```python
from build123d import *

# Parameters (mm, degrees)
CUT_EXTRUDE1_DEPTH      = 173.110429667
CUT_EXTRUDE1_DEPTH_BACK = 12.7
SKETCH2_W               = 15.5
SKETCH2_H               = 15.5


with BuildPart() as part:
    # Sketch1 → Revolve1 (revolve)
    with BuildSketch(Plane.XY, mode=Mode.PRIVATE) as revolve1_sk:
        Polygon((0, 0), (170, 0), (170, 16), (12.7, 19), (0, 19), align=None)
    revolve(revolve1_sk.sketch.rotate(Axis((0, 0, 0), (1, 0, 0)), 90), axis=Axis((0, 0, 0), (1, 0, 0)))

    # Sketch2 → Cut-Extrude1 (cut, two sides: drawn at the far end of the back side and taken through both)
    with BuildSketch(Plane(origin=(170, 0, 0), x_dir=(0, 0, -1), z_dir=(1, 0, 0)).offset(-CUT_EXTRUDE1_DEPTH_BACK)):
        Rectangle(SKETCH2_W, SKETCH2_H)
    extrude(amount=CUT_EXTRUDE1_DEPTH + CUT_EXTRUDE1_DEPTH_BACK, mode=Mode.SUBTRACT)


solid = part.part
```
Here's how the part is built. I have some questions about the finished solid (model axes, mm). A direction names the side the tool comes from. Give positions to 0.01 mm unless a question says otherwise; leave off trailing zeros. Loops run counter-clockwise (first coordinate to the right, second up) from the corner with the lowest first, then second, coordinate; pieces in that order, holes last. Notation, with made-up numbers: M 52,62.25 L 65,62.25 A25 ccw 65,77.25 Z; hole C -34,64 d7. An arc over 180 degrees is marked long. Use one line per item in the form item = value. Start each with the question number.
Q1. If we section it at B-B (x = 80): Write out the boundary of the cut face in (y, z).
Q2. I need wall thicknesses on line 1 along X through (y, z) = (-4.5, 1.5); line 2 along Z through (x, y) = (9, -1); line 3 along Y through (x, z) = (105, 11.5). Which ranges of each line are inside material? Lowest first, please.
Q3. If we section it at A-A (x = 22.5): Write out the boundary of the cut face in (y, z).
Q4. Thinking about a two-plate mould opening in Z: for faces 3 (the conical face through (90.2, -5.3, 16.7)), 4 (the flat face through (164, 0, 7.75)), 5 (the flat face through (170, 0, -10)), which applies, +Z half, -Z half, draft (parallel to the pull), parting line (faces both ways), or undercut?
Q5. Which directions (+Z, -Z, +X, -X, +Y, -Y) give clear straight access to the entire face, cutting with the end or side of a thin tool? Please do faces 1 (the flat face through (164, 7.75, 0)), 2 (the flat face through (0, 0, 0)).
Q6. Will these pins go through, and if not, where does the flat tip stop? pin 1 Ø1 at (x, y) = (136.5, -5) entering from +Z; pin 2 Ø10 at (x, y) = (161, 2) entering from -Z; pin 3 Ø12 at (x, z) = (103, -9.5) entering from +Y.
Taken from the geometry:
q1.outline = C 0,0 d35.43
q2.line_1 = 0 to 157.3
q2.line_2 = -18.97 to 18.97
q2.line_3 = -12.84 to 12.84
q3.outline = C 0,0 d37.63
q4.face_3 = parting line
q4.face_4 = undercut
q4.face_5 = draft
q5.face_1 = +X
q5.face_2 = +Z, -Z, -X, +Y, -Y
q6.pin_1 = 16.02
q6.pin_2 = -16.26
q6.pin_3 = 16.93
